Part model, mm, in its own coordinate system. Coordinates: 2 decimals unless noted, no trailing zeros. Order: outer loops, then holes, each group sorted by start corner. A loop starts at its lowest first (then second) coordinate and runs counter-clockwise, first axis right, second up.
from build123d import *

# Parameters (mm, degrees)
SKETCH1_W                    = 36
SKETCH1_H                    = 2480
BASE_FLANGE1_DEPTH           = 2
EDGE_FLANGE1_STRIP_W         = 13
EDGE_FLANGE1_STRIP_H         = 2
EDGE_FLANGE1_STRIP_CUT_DEPTH = 2480
EDGE_FLANGE1_DEPTH           = 2480
EDGE_FLANGE2_STRIP_W         = 13
EDGE_FLANGE2_STRIP_H         = 2
EDGE_FLANGE2_STRIP_CUT_DEPTH = 2480
EDGE_FLANGE2_DEPTH           = 2480
EDGE_FLANGE3_STRIP_W         = 13
EDGE_FLANGE3_STRIP_H         = 2
EDGE_FLANGE3_STRIP_CUT_DEPTH = 2480
EDGE_FLANGE3_DEPTH           = 2480
EDGE_FLANGE4_STRIP_W         = 13
EDGE_FLANGE4_STRIP_H         = 2
EDGE_FLANGE4_STRIP_CUT_DEPTH = 2480
EDGE_FLANGE4_DEPTH           = 2480
EDGE_FLANGE5_STRIP_W         = 13
EDGE_FLANGE5_STRIP_H         = 2
EDGE_FLANGE5_STRIP_CUT_DEPTH = 2480
EDGE_FLANGE5_DEPTH           = 2480
SKETCH21_R                   = 6
CUT_EXTRUDE1_DEPTH           = 10
LPATTERN1_COUNT              = 16
LPATTERN1_PITCH              = 152


# Sheet-metal steps are written as plain solids
with BuildPart() as part:
    # Sketch1 → Base-Flange1 (new body)
    with BuildSketch(Plane.XY):
        Rectangle(SKETCH1_W, SKETCH1_H)
    extrude(amount=-BASE_FLANGE1_DEPTH)

    # Edge-Flange1 strip (across the edge) → Edge-Flange1 strip cut (cut)
    with BuildSketch(Plane(origin=(-18, 1240, 0), x_dir=(1, 0, 0), z_dir=(0, -1, 0))):
        with Locations((-2, -1)):
            Rectangle(EDGE_FLANGE1_STRIP_W, EDGE_FLANGE1_STRIP_H)
    extrude(amount=EDGE_FLANGE1_STRIP_CUT_DEPTH, mode=Mode.SUBTRACT)

    # Edge-Flange1 section (across the edge) → Edge-Flange1 (add)
    with BuildSketch(Plane(origin=(-18, 1240, 0), x_dir=(1, 0, 0), z_dir=(0, -1, 0))):
        with BuildLine():
            Line((0, 2.5), (0, 13))
            Line((0, 13), (2, 13))
            Line((2, 13), (2, 2.5))
            ThreePointArc((2, 2.5), (2.732233047, 0.732233047), (4.5, 0))
            Line((4.5, 0), (4.5, -2))
            ThreePointArc((4.5, -2), (1.318019485, -0.681980515), (0, 2.5))
        make_face()
    extrude(amount=EDGE_FLANGE1_DEPTH)

    # Edge-Flange2 strip (across the edge) → Edge-Flange2 strip cut (cut)
    with BuildSketch(Plane(origin=(18, -1240, 0), x_dir=(-1, 0, 0), z_dir=(0, 1, 0))):
        with Locations((-2, -1)):
            Rectangle(EDGE_FLANGE2_STRIP_W, EDGE_FLANGE2_STRIP_H)
    extrude(amount=EDGE_FLANGE2_STRIP_CUT_DEPTH, mode=Mode.SUBTRACT)

    # Edge-Flange2 section (across the edge) → Edge-Flange2 (add)
    with BuildSketch(Plane(origin=(18, -1240, 0), x_dir=(-1, 0, 0), z_dir=(0, 1, 0))):
        with BuildLine():
            Line((0, 2.5), (0, 21))
            Line((0, 21), (2, 21))
            Line((2, 21), (2, 2.5))
            ThreePointArc((2, 2.5), (2.732233047, 0.732233047), (4.5, 0))
            Line((4.5, 0), (4.5, -2))
            ThreePointArc((4.5, -2), (1.318019485, -0.681980515), (0, 2.5))
        make_face()
    extrude(amount=EDGE_FLANGE2_DEPTH)

    # Edge-Flange3 strip (across the edge) → Edge-Flange3 strip cut (cut)
    with BuildSketch(Plane(origin=(18, 1240, 21), x_dir=(0, 0, -1), z_dir=(0, -1, 0))):
        with Locations((-2, -1)):
            Rectangle(EDGE_FLANGE3_STRIP_W, EDGE_FLANGE3_STRIP_H)
    extrude(amount=EDGE_FLANGE3_STRIP_CUT_DEPTH, mode=Mode.SUBTRACT)

    # Edge-Flange3 section (across the edge) → Edge-Flange3 (add)
    with BuildSketch(Plane(origin=(18, 1240, 21), x_dir=(0, 0, -1), z_dir=(0, -1, 0))):
        with BuildLine():
            Line((0, 2.5), (0, 48))
            Line((0, 48), (2, 48))
            Line((2, 48), (2, 2.5))
            ThreePointArc((2, 2.5), (2.732233047, 0.732233047), (4.5, 0))
            Line((4.5, 0), (4.5, -2))
            ThreePointArc((4.5, -2), (1.318019485, -0.681980515), (0, 2.5))
        make_face()
    extrude(amount=EDGE_FLANGE3_DEPTH)

    # Edge-Flange4 strip (across the edge) → Edge-Flange4 strip cut (cut)
    with BuildSketch(Plane(origin=(66, 1240, 19), x_dir=(-1, 0, 0), z_dir=(0, -1, 0))):
        with Locations((-2, -1)):
            Rectangle(EDGE_FLANGE4_STRIP_W, EDGE_FLANGE4_STRIP_H)
    extrude(amount=EDGE_FLANGE4_STRIP_CUT_DEPTH, mode=Mode.SUBTRACT)

    # Edge-Flange4 section (across the edge) → Edge-Flange4 (add)
    with BuildSketch(Plane(origin=(66, 1240, 19), x_dir=(-1, 0, 0), z_dir=(0, -1, 0))):
        with BuildLine():
            Line((0, 2.5), (0, 23))
            Line((0, 23), (2, 23))
            Line((2, 23), (2, 2.5))
            ThreePointArc((2, 2.5), (2.732233047, 0.732233047), (4.5, 0))
            Line((4.5, 0), (4.5, -2))
            ThreePointArc((4.5, -2), (1.318019485, -0.681980515), (0, 2.5))
        make_face()
    extrude(amount=EDGE_FLANGE4_DEPTH)

    # Edge-Flange5 strip (across the edge) → Edge-Flange5 strip cut (cut)
    with BuildSketch(Plane(origin=(64, 1240, -4), x_dir=(0, 0, 1), z_dir=(0, -1, 0))):
        with Locations((-2, -1)):
            Rectangle(EDGE_FLANGE5_STRIP_W, EDGE_FLANGE5_STRIP_H)
    extrude(amount=EDGE_FLANGE5_STRIP_CUT_DEPTH, mode=Mode.SUBTRACT)

    # Edge-Flange5 section (across the edge) → Edge-Flange5 (add)
    with BuildSketch(Plane(origin=(64, 1240, -4), x_dir=(0, 0, 1), z_dir=(0, -1, 0))):
        with BuildLine():
            Line((0, 2.5), (0, 13))
            Line((0, 13), (2, 13))
            Line((2, 13), (2, 2.5))
            ThreePointArc((2, 2.5), (2.732233047, 0.732233047), (4.5, 0))
            Line((4.5, 0), (4.5, -2))
            ThreePointArc((4.5, -2), (1.318019485, -0.681980515), (0, 2.5))
        make_face()
    extrude(amount=EDGE_FLANGE5_DEPTH)

    # Sketch21 → Cut-Extrude1 (cut)
    with BuildSketch(Plane.XY):
        with Locations((0, 1140)):
            Circle(SKETCH21_R)
    cut_extrude1 = extrude(amount=-CUT_EXTRUDE1_DEPTH, mode=Mode.SUBTRACT)

    # LPattern1: Cut-Extrude1 ×16
    with Locations(*[(0, -i * LPATTERN1_PITCH, 0) for i in range(1, LPATTERN1_COUNT)]):
        add(cut_extrude1, mode=Mode.SUBTRACT)


solid = part.part
Q1. Cut at A-A on y = -291. Write the cut outline in (x, z).
Results list:
outline: (-18, 2.5) arc R4.5 ccw to (-13.5, -2) - (13.5, -2) arc R4.5 ccw to (18, 2.5) - (18, 16.5) arc R2.5 cw to (20.5, 19) - (61.5, 19) arc R2.5 cw to (64, 16.5) - (64, 0.5) arc R2.5 cw to (61.5, -2) - (51, -2) - (51, -4) - (61.5, -4) arc R4.5 ccw to (66, 0.5) - (66, 16.5) arc R4.5 ccw to (61.5, 21) - (20.5, 21) arc R4.5 ccw to (16, 16.5) - (16, 2.5) arc R2.5 cw to (13.5, 0) - (-13.5, 0) arc R2.5 cw to (-16, 2.5) - (-16, 13) - (-18, 13) - close
Q2. Mould opens along X. For faces 1 (the face through (41, 17, 21)), 2 (the face through (41, 17, 19)) say: pulls with the +X half, pulls with the -X half, needs draft (parallel to the pull), parting line crosses it, or undercut.
Results list:
face 1: needs draft
face 2: undercut
Q3. Wall check: line 1 along X through (y, z) = (416, 8.25); line 2 along Z through (x, y) = (61, -932); line 3 along X through (y, z) = (-723, 17.5). Give the ranges that are in metal, low to high.
Results list:
line 1: x = -18 to -16, 16 to 18, 64 to 66
line 2: z = -4 to -2, 19 to 21
line 3: x = 16.11 to 18.21, 63.79 to 65.89
Q4. Pin check, flat tips, straight feed: pin 1 Ø15.5 at (x, y) = (0, -1140) entering from +Z; pin 2 Ø1.6 at (x, y) = (-17, -141.5) entering from +Z; pin 3 Ø1 at (y, z) = (-262, 0.5) entering from -X. Stop position of each tip, or through.
Results list:
pin 1: stops at z = 0
pin 2: stops at z = 13
pin 3: stops at x = -17.74
